Print and shaded views of the part. All mm, measured from the part's lowest x, y and z. Give positions to 0.01 mm unless a question says otherwise; leave off trailing zeros. Order: outer loops, then holes, each group sorted by start corner. A loop starts at its lowest first (then second) coordinate and runs counter-clockwise, first axis right, second up. Notation, with made-up numbers: (63, 21.5) - (118, 21.5) arc R17 cw to (118, 53.5) - close; hole circle Ø9 at (16.5, 12.25). An arc over 180 degrees is marked (long way). Answer in a Markdown table with one row per item.
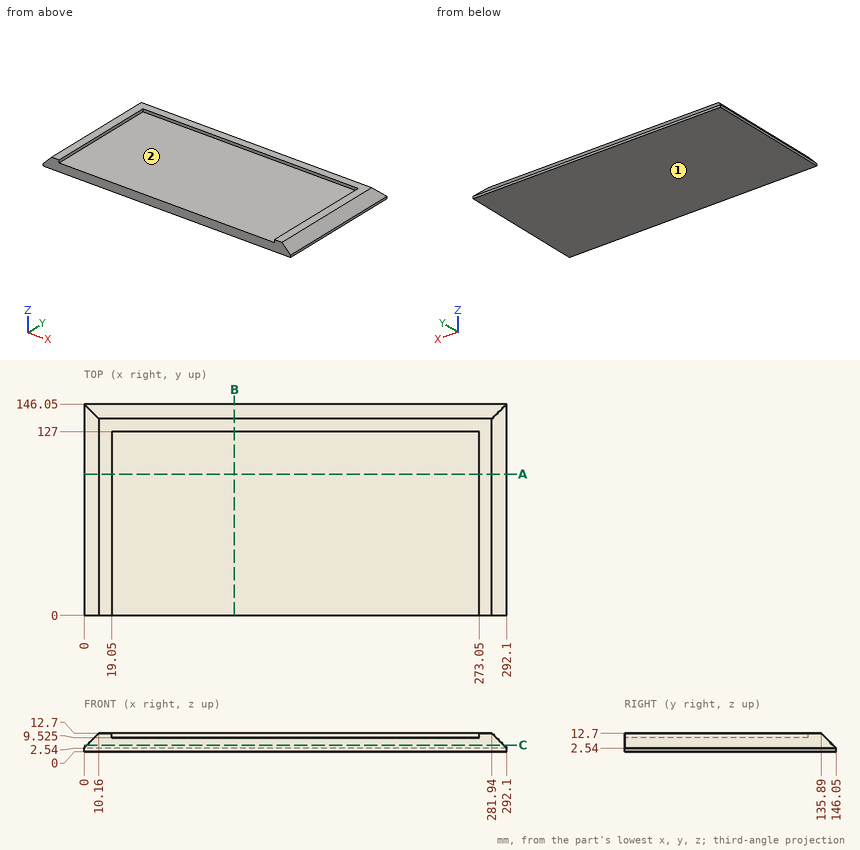
1. Cut at A-A on y = 97.5. Write the cut outline in (x, z) (3 decimals).
Check result:
| item | result |
|---|---|
| outline | (0, 0) - (292.1, 0) - (292.1, 2.54) - (281.94, 12.7) - (273.05, 12.7) - (273.05, 9.525) - (19.05, 9.525) - (19.05, 12.7) - (10.16, 12.7) - (0, 2.54) - close |
2. Cut at B-B on x = 104. Write the cut outline in (y, z) (3 decimals).
Check result:
| item | result |
|---|---|
| outline | (0, 0) - (146.05, 0) - (146.05, 2.54) - (135.89, 12.7) - (127, 12.7) - (127, 9.525) - (0, 9.525) - close |
3. Probe line 1 (Z direction, x = 229, y = 28) (3 decimals); line 2 (X direction, y = 84, z = 10.25); line 3 (X direction, y = 15, z = 10.5). List the from-to ranges inside material, lowest first.
Check result:
| item | result |
|---|---|
| line 1 | z = 0 to 9.525 |
| line 2 | x = 7.71 to 19.05, 273.05 to 284.39 |
| line 3 | x = 7.96 to 19.05, 273.05 to 284.14 |
4. Drop flat-ended pins along their axis: P1, Ø2.5, axis at y = 65.5, z = 11.5, coming from the -X side; P2, Ø2, axis at x = 108, z = 6, coming from the +Y side; P3, Ø3, axis at y = 21.5, z = 9.5, coming from the +X side. Give the stop position or say it passes through.
Check result:
| item | result |
|---|---|
| P1 | stops at x = 7.71 |
| P2 | stops at y = 143.59 |
| P3 | stops at x = 286.64 |
5. Two-plate mould, pull along X, no slides. Class the marked faces 1 and 2: +X half, -X half, draft (parallel to the pull), parting line (faces both ways), or undercut.
Check result:
| item | result |
|---|---|
| face 1 | draft |
| face 2 | undercut |
6. Cut at C-C on z = 4.5. Write the cut outline in (x, y), and give its area (3 significant figures).
Check result:
| item | result |
|---|---|
| outline | (1.96, 0) - (290.14, 0) - (290.14, 144.09) - (1.96, 144.09) - close |
| area | 41,500 mm² |
